For this review, take the finished solid that the model builds, in its own axes (mm). A direction names the side the tool comes from. Coordinates: 2 decimals unless noted, no trailing zeros. Write each loop counter-clockwise with the first axis right and the second up, starting at its lowest first coordinate (ties: lowest second). Pieces come first, ordered by that corner, then holes. Notation, with made-up numbers: (37, -37.75) -> (78, -37.75) arc R23 cw to (78, -24.75) -> close; hole circle Ø7 at (37.5, 65). An arc over 180 degrees is marked (long way). Put each result on its own line as item: value. Start each with the question number.
Item 1: To check wall thickness, follow L1, parallel to X at y = 1, z = 11.75; L2, parallel to Y at x = 0, z = 3.5; L3, parallel to Z at x = -14.5, y = 19.5. State the ranges of each line that lie inside material, in increasing order.
Item 2: Consider section A-A on y = 0. Give the boundary of the cut face in (x, z).
Item 3: The part is to be moulded in two halves that separate along Y. For faces 1 (the cylindrical face through (30.5, -12.6, 12.4)), 2 (the flat face through (0, 1, 1.5)), 3 (the flat face through (0, 0, 0)), say which applies: +Y half, -Y half, draft (parallel to the pull), parting line (faces both ways), or undercut.
Item 4: For faces 4 (the flat face through (-22, 0, 23)), 5 (the flat face through (0, -26.396, 12)), list the 3-axis set-ups (+Z, -Z, +X, -X, +Y, -Y) from which the entire face can be reached by the end or side of a thin tool; tool diameter is ignored.
Item 5: Consider section B-B on z = 9.75. Give the boundary of the cut face in (x, y), and give its area (3 significant figures).
Item 6: Insertion check: P1, Ø6.5, axis at x = -4.5, z = 15.5, coming from the -Y side; P2, Ø2, axis at y = -4, z = 10.5, coming from the -X side; P3, Ø5, axis at y = -10, z = 5, coming from the +X side. Each pin has a flat end and moves straight along its axis. Give the tip position at first contact, or say it passes through.
Item 7: Consider section C-C on x = 0. Give the boundary of the cut face in (y, z).
```python
from build123d import *

# Parameters (mm, degrees)
SKETCH_R     = 33
PAD_DEPTH    = 23
SKETCH001_W  = 30.1
SKETCH001_H  = 54.8
POCKET_DEPTH = 21.5
FILLET_R     = 2


with BuildPart() as part:
    # Sketch → Pad (new body)
    with BuildSketch(Plane.XY):
        Circle(SKETCH_R)
    extrude(amount=PAD_DEPTH)

    # Sketch001 (on Face3 of Pad) → Pocket (cut)
    with BuildSketch(Plane.XY.offset(23)):
        with Locations((0, 1.004219)):
            Rectangle(SKETCH001_W, SKETCH001_H)
    extrude(amount=-POCKET_DEPTH, mode=Mode.SUBTRACT)

    # Fillet
    fillet_edges = [part.edges().sort_by_distance(p)[0] for p in [
        (-33, 0, 0),
    ]]
    fillet(fillet_edges, radius=FILLET_R)


solid = part.part
```
Return value:
1. L1: -32.98 to -15.05, 15.05 to 32.98
1. L2: -33 to -26.4, 28.4 to 33
1. L3: 0 to 1.5
2. outline: (-33, 2) arc R2 ccw to (-31, 0) -> (31, 0) arc R2 ccw to (33, 2) -> (33, 23) -> (15.05, 23) -> (15.05, 1.5) -> (-15.05, 1.5) -> (-15.05, 23) -> (-33, 23) -> close
3. face 1: parting line
3. face 2: undercut
3. face 3: draft
4. face 4: +Z, +X, -X, +Y, -Y
4. face 5: +Z
5. outline: circle Ø66 at (0, 0); hole (-15.05, -26.4) -> (15.05, -26.4) -> (15.05, 28.4) -> (-15.05, 28.4) -> close
5. area: 1,770 mm^2
6. P1: y = -32.98
6. P2: x = -32.86
6. P3: x = 32.14
7. outline: (-33, 2) arc R2 ccw to (-31, 0) -> (31, 0) arc R2 ccw to (33, 2) -> (33, 23) -> (28.4, 23) -> (28.4, 1.5) -> (-26.4, 1.5) -> (-26.4, 23) -> (-33, 23) -> close
